Can you work these out from the model? Positions are in its coordinate system, mm. A direction names the side the tool comes from. Give positions to 0.01 mm unless a question says otherwise; leave off trailing zeros. Order: outer loops, then holes, each group sorted by start corner. A loop starts at its lowest first (then second) coordinate and runs counter-clockwise, first axis right, second up. Notation, with made-up numbers: (28.25, 44.25) -> (39.25, 44.25) arc R28 cw to (39.25, 69.25) -> close; hole circle Ø1 at (37.5, 18). An arc over 180 degrees is marked (long way). Answer as a JSON object with one key per item and string values.
```python
from build123d import *

# Parameters (mm, degrees)
BOSS_EXTRUDE1_DEPTH = 30.48
CUT_EXTRUDE1_DEPTH  = 2.54
SKETCH3_R           = 0.381
SKETCH3_R_2         = 1.27
CUT_EXTRUDE2_DEPTH  = 30.48


with BuildPart() as part:
    # Sketch1 → Boss-Extrude1 (new body)
    with BuildSketch(Plane(origin=(0, 0, 0), x_dir=(0, 0, -1), z_dir=(1, 0, 0))):
        Polygon((0, 0), (7.62, 0), (7.62, 21.59), (24.13, 21.59), (24.13, 24.13), (5.08, 24.13), (5.08, 2.54), (0, 2.54), align=None)
    extrude(amount=BOSS_EXTRUDE1_DEPTH)

    # Sketch2 → Cut-Extrude1 (cut)
    with BuildSketch(Plane(origin=(0, 24.13, 0), x_dir=(1, 0, 0), z_dir=(0, 1, 0))):
        with BuildLine():
            Line((2.254723608, 21.342486419), (2.54, 10.007156719))
            ThreePointArc((2.54, 10.007156719), (6.500958303, 10.074920649), (4.572889679, 6.614236611))
            Line((4.572889679, 6.614236611), (24.432843281, 6.9))
            ThreePointArc((24.432843281, 6.9), (23.923553898, 10.516446102), (27.54, 10.007156719))
            Line((27.54, 10.007156719), (27.54, 20.292843281))
            ThreePointArc((27.54, 20.292843281), (23.570640173, 20.2392167), (25.54, 23.686))
            Line((25.54, 23.686), (25.54, 25.581417478))
            Line((25.54, 25.581417478), (4.54, 25.84529962))
            Line((4.54, 25.84529962), (4.54, 23.686))
            ThreePointArc((4.54, 23.686), (6.176653911, 19.804017551), (2.254723608, 21.342486419))
        make_face()
    extrude(amount=-CUT_EXTRUDE1_DEPTH, mode=Mode.SUBTRACT)

    # Sketch3 → Cut-Extrude2 (cut)
    with BuildSketch(Plane(origin=(0, 24.13, 0), x_dir=(1, 0, 0), z_dir=(0, 1, 0))):
        with Locations(Location((4.54, 8.9, 0), (0, 0, 270))):
            Circle(SKETCH3_R)
        with Locations(Location((4.54, 21.4, 0), (0, 0, 270))):
            Circle(SKETCH3_R)
        with Locations(Location((25.54, 21.4, 0), (0, 0, 270))):
            Circle(SKETCH3_R)
        with Locations(Location((25.54, 8.9, 0), (0, 0, 270))):
            Circle(SKETCH3_R)
        with Locations(Location((4.54, 2.169828056, 0), (0, 0, 270))):
            Circle(SKETCH3_R_2)
        with Locations(Location((25.54, 2.169828056, 0), (0, 0, 270))):
            Circle(SKETCH3_R_2)
    extrude(amount=-CUT_EXTRUDE2_DEPTH, mode=Mode.SUBTRACT)


solid = part.part
```
1. Please list where these lines run through material, in increasing order: L1, parallel to X at y = 23.55, z = -8.9; L2, parallel to Z at x = 13, y = 3; L3, parallel to Y at x = 2, z = -12.
Worked answers:
{"L1": "0 to 4.16, 4.92 to 6.83, 23.25 to 25.16, 25.92 to 30.48", "L2": "-7.62 to -5.08", "L3": "21.59 to 24.13"}
2. Will these pins go through, and if not, where does the flat tip stop? pin 1 Ø10 at (x, y) = (13.5, 21.5) entering from +Z; pin 2 Ø4 at (x, y) = (26, 6.5) entering from -Z; pin 3 Ø5 at (x, z) = (26.5, -16) entering from -Y; pin 4 Ø4 at (x, z) = (7, -14) entering from +Y.
Worked answers:
{"pin 1": "z = -5.08", "pin 2": "z = -7.62", "pin 3": "y = 21.59", "pin 4": "through"}
3. If we section it at C-C on z = -17.5: Please give me the cut outline in (x, y), then the cut area to 3 significant figures.
Worked answers:
{"outline": "(0, 21.59) -> (2.35, 21.59) -> (2.35, 24.13) -> (0, 24.13) -> close; (27.54, 21.59) -> (30.48, 21.59) -> (30.48, 24.13) -> (27.54, 24.13) -> close", "area": "13.4 mm²"}
4. If we mould it in two halves opening along X, with no side actions, what happens to faces 1 (the face through (6.23, 22.88, -19.86)), 2 (the face through (15, 24.13, -6)), 3 (the face through (30.48, 15, -7))? For each: +X half, -X half, draft (parallel to the pull), parting line (faces both ways), or undercut.
Worked answers:
{"face 1": "undercut", "face 2": "draft", "face 3": "+X half"}
5. For faces 4 (the face through (5.8, 1.29, -2.34)), 5 (the face through (15, 2.54, -3)), 6 (the face through (28, 21.59, -16)), which set-ups out of +Z, -Z, +X, -X, +Y, -Y let a thin tool reach every point of the face, with its end or its side?
Worked answers:
{"face 4": "+Y, -Y", "face 5": "+Z, +X, -X, +Y", "face 6": "-Z, +X, -X, -Y"}
6. If we section it at B-B on x = 22: Please give me the cut outline in (y, z) (3 decimals), then the cut area to 3 significant figures.
Worked answers:
{"outline": "(0, -7.62) -> (21.59, -7.62) -> (21.59, -6.865) -> (24.13, -6.865) -> (24.13, -5.08) -> (2.54, -5.08) -> (2.54, 0) -> (0, 0) -> close", "area": "72.3 mm²"}
7. If we section it at D-D on y = 9: Please give me the cut outline in (x, z), then the cut area to 3 significant figures.
Worked answers:
{"outline": "(0, -7.62) -> (30.48, -7.62) -> (30.48, -5.08) -> (0, -5.08) -> close", "area": "77.4 mm²"}
8. If we section it at A-A on z = -8.9: Please give me the cut outline in (x, y), then the cut area to 3 significant figures.
Worked answers:
{"outline": "(0, 21.59) -> (4.16, 21.59) -> (4.16, 24.13) -> (0, 24.13) -> close; (4.92, 21.59) -> (6.83, 21.59) -> (6.83, 24.13) -> (4.92, 24.13) -> close; (23.25, 21.59) -> (25.16, 21.59) -> (25.16, 24.13) -> (23.25, 24.13) -> close; (25.92, 21.59) -> (30.48, 21.59) -> (30.48, 24.13) -> (25.92, 24.13) -> close", "area": "31.8 mm²"}
